from build123d import *

# Parameters (mm, degrees)
SKETCH1_R           = 0.675
SKETCH1_R_2         = 0.1
BOSS_EXTRUDE1_DEPTH = 1
SKETCH6_W           = 7.115524524
SKETCH6_H           = 8.894405655
BOSS_EXTRUDE5_DEPTH = 1
BOSS_EXTRUDE2_DEPTH = 1
CUT_EXTRUDE1_DEPTH  = 0.01
BOSS_EXTRUDE3_DEPTH = 0.03
BOSS_EXTRUDE4_DEPTH = 0.03


with BuildPart() as part:
    # Sketch1 → Boss-Extrude1 (new body)
    with BuildSketch(Plane.XY):
        with BuildLine():
            Line((27.8, 35.17110115), (27.8, 30.075))
            Line((27.8, 30.075), (35.799949, 30.075))
            Line((35.799949, 30.075), (35.799949, 32.885104042))
            ThreePointArc((35.799949, 32.885104042), (35.501301, 33.1851), (35.799949, 33.485095958))
            Line((35.799949, 33.485095958), (35.799949, 34.879004042))
            ThreePointArc((35.799949, 34.879004042), (35.501301, 35.179), (35.799949, 35.478995958))
            Line((35.799949, 35.478995958), (35.799949, 36.377604042))
            ThreePointArc((35.799949, 36.377604042), (35.501301, 36.6776), (35.799949, 36.977595958))
            Line((35.799949, 36.977595958), (35.799949, 37.876204042))
            ThreePointArc((35.799949, 37.876204042), (35.501301, 38.1762), (35.799949, 38.476195958))
            Line((35.799949, 38.476195958), (35.799949, 39.374804042))
            ThreePointArc((35.799949, 39.374804042), (35.501301, 39.6748), (35.799949, 39.974795958))
            Line((35.799949, 39.974795958), (35.799949, 42.575))
            Line((35.799949, 42.575), (27.8, 42.575))
            Line((27.8, 42.575), (27.8, 38.76829885))
            ThreePointArc((27.8, 38.76829885), (28.012325235, 38.680537367), (28.100299, 38.4683))
            ThreePointArc((28.100299, 38.4683), (28.012325235, 38.256062633), (27.8, 38.16830115))
            Line((27.8, 38.16830115), (27.8, 37.26969885))
            ThreePointArc((27.8, 37.26969885), (28.012325235, 37.181937367), (28.100299, 36.9697))
            ThreePointArc((28.100299, 36.9697), (28.012325235, 36.757462633), (27.8, 36.66970115))
            Line((27.8, 36.66970115), (27.8, 35.77109885))
            ThreePointArc((27.8, 35.77109885), (28.012325235, 35.683337367), (28.100299, 35.4711))
            ThreePointArc((28.100299, 35.4711), (28.012325235, 35.258862633), (27.8, 35.17110115))
        make_face()
        with Locations((29.900001, 31.200001)):
            Circle(SKETCH1_R, mode=Mode.SUBTRACT)
        with Locations((28.6512, 34.2519)):
            Circle(SKETCH1_R_2, mode=Mode.SUBTRACT)
        with Locations((31.242, 33.7312)):
            Circle(SKETCH1_R_2, mode=Mode.SUBTRACT)
        with Locations((33.700001, 31.200001)):
            Circle(SKETCH1_R, mode=Mode.SUBTRACT)
        with Locations((33.9979, 35.6362)):
            Circle(SKETCH1_R_2, mode=Mode.SUBTRACT)
        with Locations((29.4894, 37.4523)):
            Circle(SKETCH1_R_2, mode=Mode.SUBTRACT)
        with Locations((28.6766, 39.4589)):
            Circle(SKETCH1_R_2, mode=Mode.SUBTRACT)
        with Locations((28.6766, 40.1955)):
            Circle(SKETCH1_R_2, mode=Mode.SUBTRACT)
        with Locations((28.5623, 41.0718)):
            Circle(SKETCH1_R_2, mode=Mode.SUBTRACT)
        with Locations((34.417, 40.3987)):
            Circle(SKETCH1_R_2, mode=Mode.SUBTRACT)
        with Locations((35.1282, 41.0718)):
            Circle(SKETCH1_R_2, mode=Mode.SUBTRACT)
    extrude(amount=BOSS_EXTRUDE1_DEPTH)

    # Sketch6 → Boss-Extrude5 (add)
    with BuildSketch(Plane(origin=(0, 0, 0), x_dir=(-1, 0, 0), z_dir=(0, 0, -1))):
        with Locations((-31.874094547, 37.266324599)):
            Rectangle(SKETCH6_W, SKETCH6_H)
    extrude(amount=-BOSS_EXTRUDE5_DEPTH)

    # Sketch2 → Boss-Extrude2 (add)
    with BuildSketch(Plane.XY.offset(1)):
        with BuildLine():
            Line((27.81, 32.583114), (34.9935945, 32.583114))
            ThreePointArc((34.9935945, 32.583114), (35.143737614, 33.347223347), (35.789949, 33.781754006))
            Line((35.789949, 33.781754006), (35.789949, 34.579681377))
            ThreePointArc((35.789949, 34.579681377), (35.201873894, 35.179), (35.789949, 35.778318623))
            Line((35.789949, 35.778318623), (35.789949, 36.078281557))
            ThreePointArc((35.789949, 36.078281557), (35.201874074, 36.6776), (35.789949, 37.276918443))
            Line((35.789949, 37.276918443), (35.789949, 37.576882743))
            ThreePointArc((35.789949, 37.576882743), (35.201875259, 38.1762), (35.789949, 38.775517257))
            Line((35.789949, 38.775517257), (35.789949, 39.075483568))
            ThreePointArc((35.789949, 39.075483568), (35.201876085, 39.6748), (35.789949, 40.274116432))
            Line((35.789949, 40.274116432), (35.789949, 42.565))
            Line((35.789949, 42.565), (27.81, 42.565))
            Line((27.81, 42.565), (27.81, 39.067659783))
            ThreePointArc((27.81, 39.067659783), (28.39973827, 38.4683), (27.81, 37.868940217))
            Line((27.81, 37.868940217), (27.81, 37.569061725))
            ThreePointArc((27.81, 37.569061725), (28.399740212, 36.9697), (27.81, 36.370338275))
            Line((27.81, 36.370338275), (27.81, 36.070463013))
            ThreePointArc((27.81, 36.070463013), (28.3997415, 35.4711), (27.81, 34.871736987))
            Line((27.81, 34.871736987), (27.81, 32.583114))
        make_face()
    extrude(amount=BOSS_EXTRUDE2_DEPTH)

    # Sketch3 → Cut-Extrude1 (cut)
    with BuildSketch(Plane.XY.offset(2)):
        with BuildLine():
            Line((28.81, 42.777701131), (34.789949, 42.777701131))
            Line((34.789949, 42.777701131), (34.789949, 34.183114))
            ThreePointArc((34.789949, 34.183114), (34.497055781, 33.476007219), (33.789949, 33.183114))
            Line((33.789949, 33.183114), (29.81, 33.183114))
            ThreePointArc((29.81, 33.183114), (29.102893219, 33.476007219), (28.81, 34.183114))
            Line((28.81, 34.183114), (28.81, 42.777701131))
        make_face()
    extrude(amount=-CUT_EXTRUDE1_DEPTH, mode=Mode.SUBTRACT)

    # Sketch4 → Boss-Extrude3 (add)
    with BuildSketch(Plane(origin=(0, 0, 0), x_dir=(-1, 0, 0), z_dir=(0, 0, -1))):
        with BuildLine():
            Line((-35.779949, 33.694891216), (-35.779949, 33.504385914))
            ThreePointArc((-35.779949, 33.504385914), (-35.481301, 33.1851), (-35.779949, 32.865814086))
            Line((-35.779949, 32.865814086), (-35.779949, 32.676889963))
            Line((-35.779949, 32.676889963), (-35.038756119, 32.676889963))
            ThreePointArc((-35.038756119, 32.676889963), (-34.529755447, 33.185890801), (-35.038756284, 33.694891473))
            Line((-35.038756284, 33.694891473), (-35.779949, 33.694891216))
        make_face()
        with BuildLine():
            Line((-35.779949, 35.688790945), (-35.779949, 35.498285914))
            ThreePointArc((-35.779949, 35.498285914), (-35.481301, 35.179), (-35.779949, 34.859714086))
            Line((-35.779949, 34.859714086), (-35.779949, 34.670789963))
            Line((-35.779949, 34.670789963), (-35.038756119, 34.670789963))
            ThreePointArc((-35.038756119, 34.670789963), (-34.529755625, 35.179790452), (-35.038756114, 35.688790945))
            Line((-35.038756114, 35.688790945), (-35.779949, 35.688790945))
        make_face()
        with BuildLine():
            Line((-35.779949, 37.187390945), (-35.779949, 36.996885914))
            ThreePointArc((-35.779949, 36.996885914), (-35.481301, 36.6776), (-35.779949, 36.358314086))
            Line((-35.779949, 36.358314086), (-35.779949, 36.169389963))
            Line((-35.779949, 36.169389963), (-35.038756119, 36.169389963))
            ThreePointArc((-35.038756119, 36.169389963), (-34.529755625, 36.678390452), (-35.038756114, 37.187390945))
            Line((-35.038756114, 37.187390945), (-35.779949, 37.187390945))
        make_face()
        with BuildLine():
            Line((-35.779949, 38.685990945), (-35.779949, 38.495485914))
            ThreePointArc((-35.779949, 38.495485914), (-35.481301, 38.1762), (-35.779949, 37.856914086))
            Line((-35.779949, 37.856914086), (-35.779949, 37.667989963))
            Line((-35.779949, 37.667989963), (-35.038756119, 37.667989963))
            ThreePointArc((-35.038756119, 37.667989963), (-34.529755625, 38.176990452), (-35.038756114, 38.685990945))
            Line((-35.038756114, 38.685990945), (-35.779949, 38.685990945))
        make_face()
        with BuildLine():
            Line((-27.82, 37.960089963), (-27.82, 38.148907968))
            ThreePointArc((-27.82, 38.148907968), (-28.120299, 38.4683), (-27.82, 38.787692032))
            Line((-27.82, 38.787692032), (-27.82, 38.978090945))
            Line((-27.82, 38.978090945), (-28.558756031, 38.978090945))
            ThreePointArc((-28.558756031, 38.978090945), (-29.067756767, 38.469589963), (-28.559756031, 37.960089963))
            Line((-28.559756031, 37.960089963), (-27.82, 37.960089963))
        make_face()
        with BuildLine():
            Line((-27.82, 36.461489963), (-27.82, 36.650307968))
            ThreePointArc((-27.82, 36.650307968), (-28.120299, 36.9697), (-27.82, 37.289092032))
            Line((-27.82, 37.289092032), (-27.82, 37.479490946))
            Line((-27.82, 37.479490946), (-28.559755942, 37.479490946))
            ThreePointArc((-28.559755942, 37.479490946), (-29.067756767, 36.969990989), (-28.558756031, 36.461489963))
            Line((-28.558756031, 36.461489963), (-27.82, 36.461489963))
        make_face()
        with BuildLine():
            Line((-35.779949, 40.184590945), (-35.779949, 39.994085914))
            ThreePointArc((-35.779949, 39.994085914), (-35.481301, 39.6748), (-35.779949, 39.355514086))
            Line((-35.779949, 39.355514086), (-35.779949, 39.166589963))
            Line((-35.779949, 39.166589963), (-35.038756119, 39.166589963))
            ThreePointArc((-35.038756119, 39.166589963), (-34.529755625, 39.675590452), (-35.038756114, 40.184590945))
            Line((-35.038756114, 40.184590945), (-35.779949, 40.184590945))
        make_face()
        with BuildLine():
            Line((-27.82, 34.962889963), (-27.82, 35.151707968))
            ThreePointArc((-27.82, 35.151707968), (-28.120299, 35.4711), (-27.82, 35.790492032))
            Line((-27.82, 35.790492032), (-27.82, 35.980890945))
            Line((-27.82, 35.980890945), (-28.558756031, 35.980890945))
            ThreePointArc((-28.558756031, 35.980890945), (-29.067756767, 35.472389963), (-28.559756031, 34.962889963))
            Line((-28.559756031, 34.962889963), (-27.82, 34.962889963))
        make_face()
    extrude(amount=BOSS_EXTRUDE3_DEPTH)

    # Sketch5 → Boss-Extrude4 (add)
    with BuildSketch(Plane.XY.offset(1)):
        with BuildLine():
            Line((35.799949, 39.374804042), (35.799949, 39.075363253))
            ThreePointArc((35.799949, 39.075363253), (35.20186173, 39.6748), (35.799949, 40.274236747))
            Line((35.799949, 40.274236747), (35.799949, 39.974795958))
            ThreePointArc((35.799949, 39.974795958), (35.501301, 39.6748), (35.799949, 39.374804042))
        make_face()
        with BuildLine():
            Line((27.8, 39.067738195), (27.8, 38.76829885))
            ThreePointArc((27.8, 38.76829885), (28.100299, 38.4683), (27.8, 38.16830115))
            Line((27.8, 38.16830115), (27.8, 37.868861805))
            ThreePointArc((27.8, 37.868861805), (28.39973827, 38.4683), (27.8, 39.067738195))
        make_face()
        with BuildLine():
            Line((35.799949, 37.876204042), (35.799949, 37.576763253))
            ThreePointArc((35.799949, 37.576763253), (35.20186173, 38.1762), (35.799949, 38.775636747))
            Line((35.799949, 38.775636747), (35.799949, 38.476195958))
            ThreePointArc((35.799949, 38.476195958), (35.501301, 38.1762), (35.799949, 37.876204042))
        make_face()
        with BuildLine():
            Line((35.799949, 36.377604042), (35.799949, 36.078163253))
            ThreePointArc((35.799949, 36.078163253), (35.20186173, 36.6776), (35.799949, 37.277036747))
            Line((35.799949, 37.277036747), (35.799949, 36.977595958))
            ThreePointArc((35.799949, 36.977595958), (35.501301, 36.6776), (35.799949, 36.377604042))
        make_face()
        with BuildLine():
            Line((35.799949, 34.879004042), (35.799949, 34.579563253))
            ThreePointArc((35.799949, 34.579563253), (35.20186173, 35.179), (35.799949, 35.778436747))
            Line((35.799949, 35.778436747), (35.799949, 35.478995958))
            ThreePointArc((35.799949, 35.478995958), (35.501301, 35.179), (35.799949, 34.879004042))
        make_face()
        with BuildLine():
            Line((35.799949, 32.885104042), (35.799949, 32.585663253))
            ThreePointArc((35.799949, 32.585663253), (35.20186173, 33.1851), (35.799949, 33.784536747))
            Line((35.799949, 33.784536747), (35.799949, 33.485095958))
            ThreePointArc((35.799949, 33.485095958), (35.501301, 33.1851), (35.799949, 32.885104042))
        make_face()
        with BuildLine():
            Line((27.8, 35.168301), (27.8, 34.868861805))
            ThreePointArc((27.8, 34.868861805), (28.399438195, 35.4683), (27.8, 36.067738195))
            Line((27.8, 36.067738195), (27.8, 35.768299))
            ThreePointArc((27.8, 35.768299), (28.099999, 35.4683), (27.8, 35.168301))
        make_face()
        with BuildLine():
            Line((27.8, 36.668301), (27.8, 36.368861805))
            ThreePointArc((27.8, 36.368861805), (28.399438195, 36.9683), (27.8, 37.567738195))
            Line((27.8, 37.567738195), (27.8, 37.268299))
            ThreePointArc((27.8, 37.268299), (28.099999, 36.9683), (27.8, 36.668301))
        make_face()
    extrude(amount=BOSS_EXTRUDE4_DEPTH)


solid = part.part
Geometry check sheet. Reference: the model listing, model coordinates, mm. A direction names the side the tool comes from. Give positions to 0.01 mm unless a question says otherwise; leave off trailing zeros. Order: outer loops, then holes, each group sorted by start corner. A loop starts at its lowest first (then second) coordinate and runs counter-clockwise, first axis right, second up. Notation, with made-up numbers: M 11,83.25 L 32,83.25 A18 ccw 32,91.25 Z; hole C 55,77 d11. An arc over 180 degrees is marked long. Use a Markdown table: item, result.
Item 1: Draft check along X on faces 1 (the cylindrical face through (30.26, 31.77, 0.49)), 2 (the flat face through (35.8, 38.9, 0.5)), 3 (the flat face through (31.4, 32.583, 1.5)). Enter one of: +X half, -X half, draft (parallel to the pull), parting line (faces both ways), or undercut.
Answers follow:
| item | result |
|---|---|
| face 1 | undercut |
| face 2 | +X half |
| face 3 | draft |
Item 2: Material ranges on line 1 along Y through (x, z) = (33.7, 0.4) (3 decimals); line 2 along Y through (x, z) = (35.75, 1.3) (3 decimals); line 3 along Y through (x, z) = (32.75, 1.35) (3 decimals), recorded low to high.
Answers follow:
| item | result |
|---|---|
| line 1 | y = 30.075 to 30.525, 31.875 to 42.575 |
| line 2 | y = 33.773 to 34.582, 35.776 to 36.08, 37.275 to 37.579, 38.773 to 39.078, 40.272 to 42.565 |
| line 3 | y = 32.583 to 42.565 |
Item 3: Tool access check on faces 4 (the flat face through (31.9, 42.565, 1.5)), 5 (the cylindrical face through (35.202, 36.665, 1.508)), 6 (the flat face through (32, 38, 1.99)). Record the directions out of +Z, -Z, +X, -X, +Y, -Y that give a thin tool (end or side, any length) a straight path to the whole face; none if there is none.
Answers follow:
| item | result |
|---|---|
| face 4 | +Z, +X, -X, +Y |
| face 5 | +Z, +X |
| face 6 | +Z, +Y |
Item 4: Section check D-D (x = 32.5). Record the cut outline in (y, z) (3 decimals).
Answers follow:
| item | result |
|---|---|
| outline | M 30.075,0 L 42.575,0 L 42.575,1 L 42.565,1 L 42.565,1.99 L 33.183,1.99 L 33.183,2 L 32.583,2 L 32.583,1 L 30.075,1 Z |
Item 5: Section check C-C (z = 1.6). Record the cut outline in (x, y) (3 decimals).
Answers follow:
| item | result |
|---|---|
| outline | M 27.81,32.583 L 34.994,32.583 A1.018 cw 35.79,33.782 L 35.79,34.58 A0.599 cw 35.79,35.778 L 35.79,36.078 A0.599 cw 35.79,37.277 L 35.79,37.577 A0.599 cw 35.79,38.776 L 35.79,39.075 A0.599 cw 35.79,40.274 L 35.79,42.565 L 27.81,42.565 L 27.81,39.068 A0.599 cw 27.81,37.869 L 27.81,37.569 A0.599 cw 27.81,36.37 L 27.81,36.07 A0.599 cw 27.81,34.872 Z |
Item 6: Depth check by flat-ended pin: P1, Ø0.8, axis at y = 41, z = 1.5, coming from the -X side; P2, Ø2, axis at x = 30.5, y = 34, coming from the -Z side. Enter the tip coordinate at first touch or a pass-through.
Answers follow:
| item | result |
|---|---|
| P1 | stops at x = 27.81 |
| P2 | stops at z = 0 |
Item 7: Section check A-A (x = 34). Record the cut outline in (y, z) (3 decimals), and give its area (3 significant figures).
Answers follow:
| item | result |
|---|---|
| outline | M 30.075,0 L 30.595,0 L 30.595,1 L 30.075,1 Z; M 31.805,0 L 42.575,0 L 42.575,1 L 42.565,1 L 42.565,1.99 L 33.205,1.99 L 33.205,2 L 32.583,2 L 32.583,1 L 31.805,1 Z |
| area | 21.2 mm2 |
